```python
from build123d import *

# Parameters (mm, degrees)
F3_DEPTH = 12.7


with BuildPart() as f1:
    # F0 (on Front) → F1 (revolve)
    with BuildSketch(Plane.XZ):
        Polygon((-153.5377800465, 190.3918104444), (-35.5008375951, 18.8378337771), (-31.2896880625, 18.8378337771), (-149.1814106703, 191.8626129627), align=None)
        Polygon((-35.5008375951, 18.8378337771), (-22.5395507474, 0), (-18.4543896466, 0), (-31.2896880625, 18.8378337771), align=None)
    revolve(axis=Axis((-32.7495573248, 0, 110.0577637553), (-0.2852077577, 0, 0.9584657192)))

    # F2 (on Top) → F3 (join, symmetric)
    with BuildSketch(Plane.XY):
        with BuildLine():
            Line((-39.649366063, -86.1673603178), (46.5179942548, 0))
            Line((46.5179942548, 0), (18.8556073768, 0))
            ThreePointArc((18.8556073768, 0), (0, -18.8556073768), (-18.8556073768, 0))
            Line((-18.8556073768, 0), (-39.649366063, 0))
            Line((-39.649366063, 0), (-39.649366063, -86.1673603178))
        make_face()
        with BuildLine():
            Line((18.8556073768, 0), (46.5179942548, 0))
            Line((46.5179942548, 0), (-39.649366063, 86.1673603178))
            Line((-39.649366063, 86.1673603178), (-39.649366063, 0))
            Line((-39.649366063, 0), (-18.8556073768, 0))
            ThreePointArc((-18.8556073768, 0), (0, 18.8556073768), (18.8556073768, 0))
        make_face()
    extrude(amount=F3_DEPTH, both=True)


solid = f1.part
```
Geometry check sheet. Reference: the model listing, model coordinates, mm. A direction names the side the tool comes from. Round coordinates to 2 decimals unless told otherwise and drop trailing zeros. Use a Markdown table: item, result. Add a question column.
(1) Release check for a two-part mould opening along Z. For faces 6 (the flat face through (2.83, -43.69, 0.18)), 7 (the flat face through (-19, -1, 12.7)), 8 (the flat face through (-35, 1, 12.7)) record: pulls with the +Z half, pulls with the -Z half, needs draft (parallel to the pull), parting line crosses it, or undercut.
(2) Tool access check on faces 1 (the flat face through (-39.649, 1, 0)), 2 (the flat face through (4.04, 42.48, 0.18)), 3 (the conical face through (-145.53, -26.6, 192.94)), 4 (the flat face through (-26, 1, -12.7)), 5 (the cylindrical face through (-18.85, -0.45, 8.07)). Record the directions out of +Z, -Z, +X, -X, +Y, -Y that give a thin tool (end or side, any length) a straight path to the whole face; none if there is none.
(3) Material ranges on line 1 along X through (y, z) = (0, 4); line 2 along Z through (x, y) = (-22, -25.5); line 3 along Y through (x, z) = (0, -5), recorded low to high. Write a range as [from, to].
(4) Depth check by flat-ended pin: pin 1 (7.5 mm diameter, centred on y = 12.5, z = -1.5, fed in from -X); pin 2 (1.5 mm diameter, centred on y = -31, z = 45, fed in from -X); pin 3 (12 mm diameter, centred on y = 56, z = 120.5, fed in from +X). Enter the tip coordinate at first touch or a pass-through.
Answers below:
| question | item | result |
|---|---|---|
| 1 | face 6 | needs draft |
| 1 | face 7 | pulls with the +Z half |
| 1 | face 8 | undercut |
| 2 | face 1 | -Z, -X, +Y, -Y |
| 2 | face 2 | -Z, +X, +Y |
| 2 | face 3 | +Z, -X |
| 2 | face 4 | -Z, +X, -X, +Y, -Y |
| 2 | face 5 | +Z |
| 3 | line 1 | [-39.65, -18.86], [18.86, 46.52] |
| 3 | line 2 | [-12.7, 12.7], [24.44, 32.86] |
| 3 | line 3 | [-46.52, -18.86], [18.86, 46.52] |
| 4 | pin 1 | x = -39.65 |
| 4 | pin 2 | x = -35.37 |
| 4 | pin 3 | x = -6.01 |
